Part print with two shaded views. Sizes in mm from the minimum x, y, z corner. A direction names the side the tool comes from. Coordinates: 2 decimals unless noted, no trailing zeros. Loops run counter-clockwise (first coordinate to the right, second up) from the corner with the lowest first, then second, coordinate; pieces in that order, holes last.
Item 1: Drill centre lines: line 1 along Y through (x, z) = (4.25, 1.35); line 2 along X through (y, z) = (1.75, 1.35). Where is each one in solid material? Low to high.
Item 2: 3-axis set-ups, long thin cutter, end or side, ignore diameter. For the marked faces 4, 5 and 6: which of +Z, -Z, +X, -X, +Y, -Y reach the whole face in a straight line?
Item 3: Mould opens along X. For the marked faces 1, 2 and 3 say: released by +X, released by -X, zero draft, split by the parting line, or undercut.
Item 4: Cut at A-A (z = 0.9). List the corners of the cut face in (x, y).
Item 5: Cut at C-C (x = 4.5). List the corners of the cut face in (y, z).
Item 6: Cut at B-B (y = 2.75). List the corners of the cut face in (x, z).
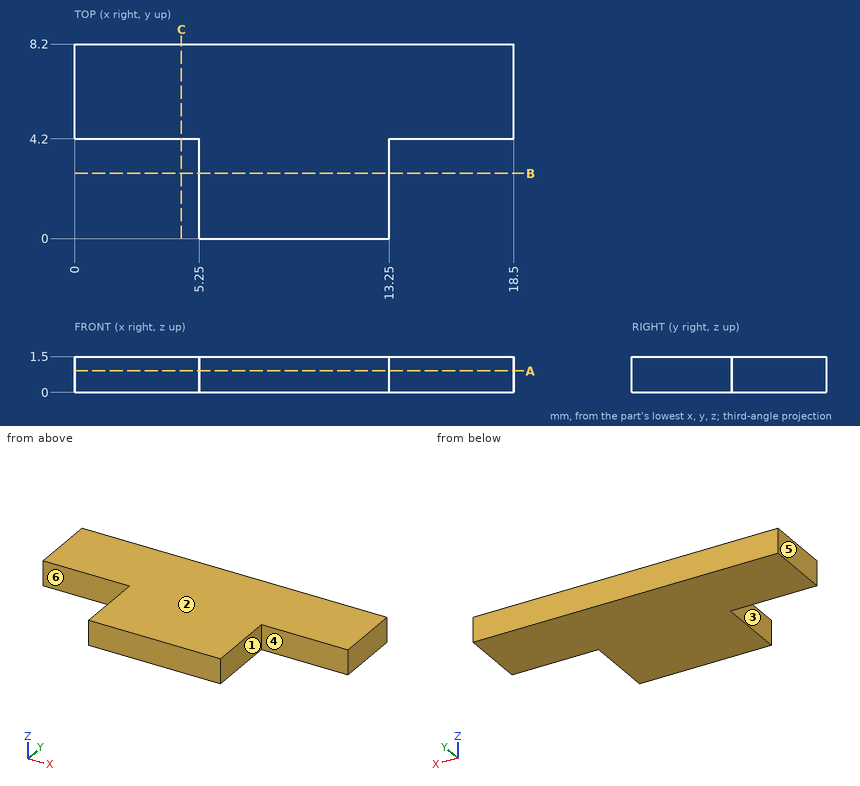
Filled sheet:
1. line 1: y = 4.2 to 8.2
1. line 2: x = 5.25 to 13.25
2. face 4: +Z, -Z, +X, -Y
2. face 5: +Z, -Z, -X, +Y, -Y
2. face 6: +Z, -Z, -X, -Y
3. face 1: released by +X
3. face 2: zero draft
3. face 3: released by -X
4. outline: (0, 4.2) - (5.25, 4.2) - (5.25, 0) - (13.25, 0) - (13.25, 4.2) - (18.5, 4.2) - (18.5, 8.2) - (0, 8.2) - close
5. outline: (4.2, 0) - (8.2, 0) - (8.2, 1.5) - (4.2, 1.5) - close
6. outline: (5.25, 0) - (13.25, 0) - (13.25, 1.5) - (5.25, 1.5) - close
